from build123d import *

# Parameters (mm, degrees)
F0_W     = 38.1
F0_H     = 25.4
F1_DEPTH = 12.7
F3_DEPTH = 19.05
F2_W     = 12.660892
F2_H     = 12.70006
F4_DEPTH = 25.401
F6_DEPTH = 25.4
F8_DEPTH = 38.101


with BuildPart() as f1:
    # F0 (on Front) → F1 (new body, symmetric)
    with BuildSketch(Plane.XZ):
        with Locations((19.05, 12.7)):
            Rectangle(F0_W, F0_H)
    extrude(amount=F1_DEPTH, both=True)

    # F2 (on face) → F3 (cut)
    with BuildSketch(Plane.XZ.offset(12.7)):
        Polygon((25.360892, 12.69994), (12.7, 12.69994), (12.7, 0), (25.4, 0), align=None)
    extrude(amount=-F3_DEPTH, mode=Mode.SUBTRACT)

    # F2 (on face) → F4 (cut, through all)
    with BuildSketch(Plane.XZ.offset(12.7)):
        with Locations((19.030446, 19.04997)):
            Rectangle(F2_W, F2_H)
        Polygon((12.7, 25.4), (0, 25.4), (0, 12.7), (12.7, 12.69994), align=None)
    extrude(amount=-F4_DEPTH, mode=Mode.SUBTRACT)

    # F5 (on face) → F6 (cut)
    with BuildSketch(Plane(origin=(0, 0, 0), x_dir=(0, -1, 0), z_dir=(-1, 0, 0))):
        Polygon((12.7, 12.7), (0, 12.7), (12.7, 0), align=None)
    extrude(amount=-F6_DEPTH, mode=Mode.SUBTRACT)

    # F7 (on face) → F8 (cut, through all)
    with BuildSketch(Plane.YZ.offset(38.1)):
        Polygon((-12.7, 12.7), (0, 25.4), (-12.7, 25.4), align=None)
    extrude(amount=-F8_DEPTH, mode=Mode.SUBTRACT)


solid = f1.part
Can you work these out from the model? Positions are in its coordinate system, mm. A direction names the side the tool comes from. Give positions to 0.01 mm unless a question says otherwise; leave off trailing zeros. Loops run counter-clockwise (first coordinate to the right, second up) from the corner with the lowest first, then second, coordinate; pieces in that order, holes last. Notation, with made-up numbers: M 62.5,20.25 L 96.5,20.25 A28 ccw 96.5,51.25 Z; hole C -28.75,-38 d11. An arc over 180 degrees is marked long. One line per item, written item: value.
1) I'm going to push flat-ended pins straight in: pin 1 (3 mm diameter, centred on x = 19.5, y = 9.5, fed in from +Z); pin 2 (1 mm diameter, centred on x = 26, y = -2.5, fed in from +Z); pin 3 (14 mm diameter, centred on y = -1.5, z = 19.5, fed in from -X); pin 4 (10 mm diameter, centred on y = -6, z = 22, fed in from -X). Where does each tip first touch, or does it pass through?
Geometry check:
pin 1: stops at z = 12.7
pin 2: stops at z = 23.4
pin 3: stops at x = 0
pin 4: stops at x = 25.36
2) Thinking about a two-plate mould opening in X: for faces 1 (the face through (12.7, -1, 5)), 2 (the face through (25.361, 3, 19)), 3 (the face through (19, 8, 0)), which applies, +X half, -X half, draft (parallel to the pull), parting line (faces both ways), or undercut?
Geometry check:
face 1: undercut
face 2: -X half
face 3: draft
3) Imagine slicing it at B-B on y = 11. Write out the boundary of the cut face in (x, z).
Geometry check:
outline: M 0,0 L 38.1,0 L 38.1,25.4 L 25.36,25.4 L 25.36,12.7 L 12.7,12.7 L 0,12.7 Z
4) Imagine slicing it at D-D on x = 33. Write out the boundary of the cut face in (y, z), and give its area (3 significant figures).
Geometry check:
outline: M -12.7,0 L 12.7,0 L 12.7,25.4 L 0,25.4 L -12.7,12.7 Z
area: 565 mm²
5) On a 3-axis mill with a long thin cutter (end or side, diameter ignored), from which of +Z, -Z, +X, -X, +Y, -Y can I reach the whole of each face in a straight line? I mean faces 4 (the face through (6.3, -6.3, 6.4)), 5 (the face through (19, 6.35, 6)). Say none if no direction works.
Geometry check:
face 4: +Z, -X, -Y
face 5: +Z, -Z, -Y
6) Please list where these lines run through material, in increasing order: line 1 (X direction, y = -8.5, z = 1); line 2 (Y direction, x = 19, z = 11.25); line 3 (X direction, y = 0.75, z = 16.5).
Geometry check:
line 1: x = 0 to 12.7, 25.4 to 38.1
line 2: y = 6.35 to 12.7
line 3: x = 25.36 to 38.1
